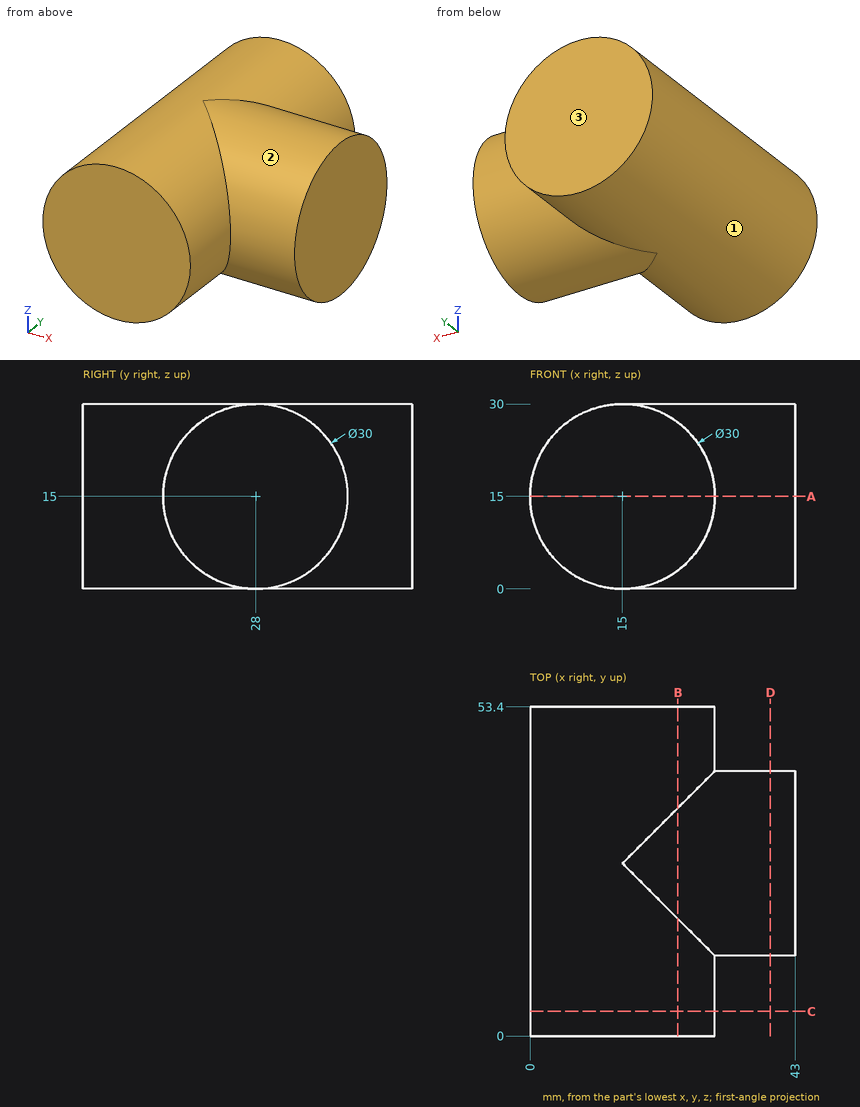
For this review, use the dimensioned drawing (mm, ordinates from the lowest corner) and the shaded views. A direction names the side the tool comes from. Coordinates: 2 decimals unless noted, no trailing zeros. Loops run counter-clockwise (first coordinate to the right, second up) from the corner with the lowest first, then second, coordinate; pieces in that order, holes last. Notation, with made-up numbers: (75, 83) - (110, 83) arc R30 cw to (110, 105) - close; hole circle Ø6 at (2.25, 32.5). An arc over 180 degrees is marked (long way). Use one line per item in the form item = value. Start each with the question number.
1) For the marked faces 1, 2 and 3, list the 3-axis set-ups (+Z, -Z, +X, -X, +Y, -Y) from which the entire face can be reached by the end or side of a thin tool; tool diameter is ignored.
2) To check wall thickness, follow probe 1 along Z at (x, y) = (5, 4); probe 2 along Z at (x, y) = (19, 27.5); probe 3 along Y at (x, z) = (38, 5.75). State the ranges of each line that lie inside material, in increasing order. Write a range as from..to.
3) Take a section at D-D (x = 39). State the section outline as (y, z) points.
4) Take a section at B-B (x = 24). State the section outline as (y, z) points, plus the area to 3 significant figures.
5) Take a section at C-C (y = 4). State the section outline as (x, z) points.
6) Take a section at A-A (z = 15). State the section outline as (x, y) points.
7) For pin 1 (6 mm diameter, centred on y = 27.5, z = 21, fed in from -X); pin 2 (2 mm diameter, centred on x = 16.5, y = 20, fed in from -Z); pin 3 (2 mm diameter, centred on x = 21.5, y = 16.5, fed in from -Z), all flat-tipped, find the tip position at first contact; note any pin that passes through.
From the geometry:
q1.face_1 = none
q1.face_2 = +X
q1.face_3 = +Z, -Z, +X, -X, +Y
q2.probe_1 = 3.82..26.18
q2.probe_2 = 0.01..29.99
q2.probe_3 = 16.19..39.81
q3.outline = circle Ø30 at (28, 15)
q4.outline = (0, 3) - (19, 3) arc R15 ccw to (37, 3) - (53.4, 3) - (53.4, 27) - (37, 27) arc R15 ccw to (19, 27) - (0, 27) - close
q4.area = 1,360 mm2
q5.outline = circle Ø30 at (15, 15)
q6.outline = (0, 0) - (30, 0) - (30, 13) - (43, 13) - (43, 43) - (30, 43) - (30, 53.4) - (0, 53.4) - close
q7.pin_1 = 0.3
q7.pin_2 = 0.01
q7.pin_3 = 1.04
